```python
from build123d import *

# Parameters (mm, degrees)
F0_R     = 11.1125
F1_DEPTH = 3.175


with BuildPart() as f1:
    # F0 (on Top) → F1 (new body)
    with BuildSketch(Plane.XY):
        Circle(F0_R)
        with BuildLine():
            ThreePointArc((1.5875, 6.148361), (5.020116, 3.888565), (6.35, 0))
            ThreePointArc((6.35, 0), (-3.888565, -5.020116), (-1.5875, 6.148361))
            Line((-1.5875, 6.148361), (-1.5875, 6.35))
            Line((-1.5875, 6.35), (-1.5875, 7.9375))
            Line((-1.5875, 7.9375), (1.5875, 7.9375))
            Line((1.5875, 7.9375), (1.5875, 6.35))
            Line((1.5875, 6.35), (1.5875, 6.148361))
        make_face(mode=Mode.SUBTRACT)
    extrude(amount=F1_DEPTH)


solid = f1.part
```
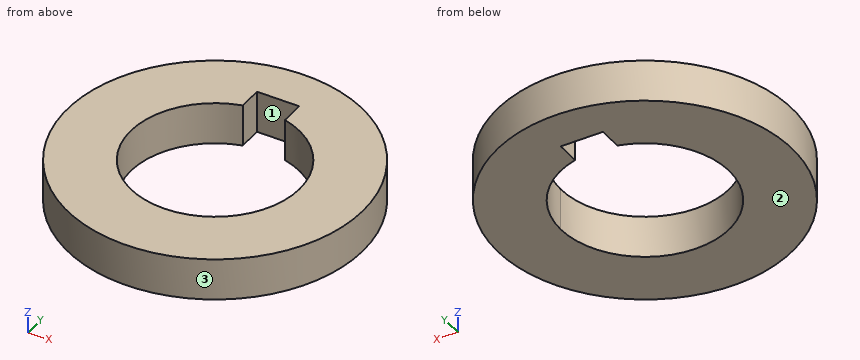
The listing builds one solid part. Answer for the finished solid, in the listing's coordinates (mm). Face numbers are marked on the shaded views. Coordinates: 2 decimals unless noted, no trailing zeros. Loops run counter-clockwise (first coordinate to the right, second up) from the corner with the lowest first, then second, coordinate; pieces in that order, holes last. Notation, with made-up numbers: (-14.5, 31.5) - (-5.5, 31.5) arc R26 cw to (-5.5, 47.5) - close; hole circle Ø9 at (10.5, 65). An arc over 180 degrees is marked (long way). Use a Markdown table: item, result. Add a question column.
1) Given pin 1 (1.5 mm diameter, centred on x = -1, z = 1.5, fed in from -Y); pin 2 (1.4 mm diameter, centred on y = 7.5, z = 1, fed in from +X); pin 3 (0.9 mm diameter, centred on y = 7, z = 2, fed in from -X), each flat-ended and moving along its own axis, determine where each tip first touches the part or whether it passes through.
2) The mould has two halves that part along X. Classify the marked faces 1, 2 and 3: released by +X, released by -X, zero draft, split by the parting line, or undercut.
3) The part is cut by section D-D, the plane x = -7. Give the vertices of the cut face in (y, z) (3 decimals).
4) Find the intervals of material crossed by line 1 (Y direction, x = 0, z = 1.35); line 2 (Y direction, x = -4, z = 2.8); line 3 (X direction, y = -1.5, z = 0.5), in increasing order.
5) The part is cut by section B-B, the plane y = 4.5. Give the vertices of the cut face in (x, z) (3 decimals).
Here are the results:
| question | item | result |
|---|---|---|
| 1 | pin 1 | stops at y = -11.11 |
| 1 | pin 2 | stops at x = 8.79 |
| 1 | pin 3 | stops at x = -8.98 |
| 2 | face 1 | undercut |
| 2 | face 2 | zero draft |
| 2 | face 3 | split by the parting line |
| 3 | outline | (-8.631, 0) - (8.631, 0) - (8.631, 3.175) - (-8.631, 3.175) - close |
| 4 | line 1 | y = -11.11 to -6.35, 7.94 to 11.11 |
| 4 | line 2 | y = -10.37 to -4.93, 4.93 to 10.37 |
| 4 | line 3 | x = -11.01 to -6.17, 6.17 to 11.01 |
| 5 | outline | (-10.161, 0) - (-4.48, 0) - (-4.48, 3.175) - (-10.161, 3.175) - close; (4.48, 0) - (10.161, 0) - (10.161, 3.175) - (4.48, 3.175) - close |
